Build history of the part. All positions in model axes, mm. Face numbers are marked on the shaded views. A direction names the side the tool comes from. Round coordinates to 2 decimals unless told otherwise and drop trailing zeros. Order: outer loops, then holes, each group sorted by start corner. A loop starts at its lowest first (then second) coordinate and runs counter-clockwise, first axis right, second up. Notation, with made-up numbers: M 50.25,11 L 97.25,11 A7 cw 97.25,16 Z; hole C 29,81 d5. An arc over 180 degrees is marked long. One line per item, written item: value. Start each with the question number.
Item 1: Band-saw the part on B-B, the plane y = -21.75. Write the cut outline in (x, z).
Item 2: Probe L1, parallel to X at y = -23.5, z = 0.7; L2, parallel to Y at x = 16.5, z = 0.6; L3, parallel to Y at x = 11, z = 0.35. List the from-to ranges inside material, lowest first.
Item 3: Band-saw the part on D-D, the plane x = 10.5. Write the cut outline in (y, z).
Item 4: Two-plate mould, pull along X, no slides. Class the marked faces 4, 5, 6 and 7: +X half, -X half, draft (parallel to the pull), parting line (faces both ways), or undercut.
Item 5: Tool access for the marked faces 1, 2 and 3: list every direction of +Z, -Z, +X, -X, +Y, -Y with a clear straight run to the whole face (end or side of a thin tool).
Item 6: Pin check, flat tips, straight feed: pin 1 (1 mm diameter, centred on x = 19, y = -35, fed in from -Z); pin 2 (2 mm diameter, centred on x = 12, y = -28.5, fed in from -Z); pin 3 (2 mm diameter, centred on y = -27.5, z = 0.5, fed in from -X). Stop position of each tip, or through.
Item 7: Band-saw the part on C-C, the plane x = 19. Write the cut outline in (y, z), then the cut area to 3 significant figures.
Item 8: Band-saw the part on A-A, the plane z = 0.8. Write the cut outline in (x, y).
Autodesk Inventor part; units mm, degrees
ref_plane "YZ Plane" through (0, 0, 0) normal (1, 0, 0) x (0, 1, 0)
ref_plane "XZ Plane" through (0, 0, 0) normal (0, 1, 0) x (-1, 0, 0)
ref_plane "XY Plane" through (0, 0, 0) normal (0, 0, 1) x (1, 0, 0)
ref_plane "Arbeitsebene1" through (0, 0, 0) normal (0, 0, 1) x (1, 0, 0)
sketch "Skizze1" plane through (0, 0, 0) normal (0, 0, 1) x (1, 0, 0)
  line L0 (8.8222, -7.25) -> (-9.1, -7.25)
  line L1 (-9.1, -7.25) -> (-9.1, 29.75)
  line L2 (-9.1, 29.75) -> (45.9, 29.75)
  line L3 (45.9, 29.75) -> (45.9, -7.25)
  line L4 (45.9, -7.25) -> (27.9778, -7.25)
  line L5 (-63.9, -32.5058) -> (-63.9, -38.75)
  line L6 (63.9, -38.75) -> (63.9, 3.9837)
  line L7 (63.9, 3.9837) -> (56.9, 3.9837)
  line L8 (56.9, 3.9837) -> (56.9, 8.0046)
  spline S0 degree 2 poles (56.9, 8.0046) (47.4544, 9.25) (56.9, 10.4954) knots 0.408689 0.408689 0.408689 2.009633 2.009633 2.009633 weights 1.06106 1.156332 1.06106
  line L9 (56.9, 10.4954) -> (56.9, 14.5163)
  line L10 (56.9, 14.5163) -> (63.9, 14.5163)
  arc A0 (63.9, 38.75) -> (59.9, 42.75) centre (59.9, 38.75) ccw
  line L11 (59.9, 42.75) -> (-59.9, 42.75)
  arc A1 (-59.9, 42.75) -> (-63.9, 38.75) centre (-59.9, 38.75) ccw
  line L12 (-63.9, 25.4963) -> (-55.9, 25.4963)
  line L13 (-55.9, 25.4963) -> (-55.9, 19.75)
  line L14 (-55.9, 19.75) -> (-18.9, 19.75)
  line L15 (-18.9, 19.75) -> (-18.9, 10.3274)
  spline S1 degree 2 poles (-18.9, 10.3274) (-11.6855, 9.25) (-18.9, 8.1726) knots 0.06387 0.06387 0.06387 0.952272 0.952272 0.952272 weights 1.010578 1.079212 1.010578
  line L16 (-18.9, 8.1726) -> (-18.9, -1.25)
  line L17 (-18.9, -1.25) -> (-55.9, -1.25)
  line L18 (-55.9, -1.25) -> (-55.9, -6.9963)
  line L19 (-55.9, -6.9963) -> (-63.9, -6.9963)
  line L20 (-63.9, -6.9963) -> (-63.9, -22.9942)
  line L21 (14.75, -32.05) -> (21.15, -32.05)
  line L22 (21.15, -32.05) -> (21.15, -24.25)
  line L23 (21.15, -24.25) -> (14.75, -24.25)
  line L24 (14.75, -24.25) -> (14.75, -32.05)
  line L25 (8.8222, -20.5) -> (30.4914, -20.5)
  line L26 (30.4914, -20.5) -> (30.4914, -39.25)
  line L27 (30.4914, -39.25) -> (8.8222, -39.25)
  line L28 (8.8222, -39.25) -> (8.8222, -20.5)
  line L29 (63.9, 14.5163) -> (63.9, 38.75)
  circle A2 centre (5.4922, -12.0867) radius 1.4
  circle A3 centre (17.95, -36.25) radius 1.4
  circle A4 centre (-27.8589, -14.9953) radius 1.4
  circle A5 centre (-42.2276, -36.25) radius 1.4
  circle A6 centre (-42.2276, -19.25) radius 1.4
  circle A7 centre (-27.8589, -39.949) radius 1.4
  circle A8 centre (27.4914, -28.65) radius 1.4
  circle A9 centre (32.285, -12.0867) radius 1.4
  line L30 (-8.36, -23.75) -> (8.8222, -23.75)
  line L31 (8.8222, -23.75) -> (8.8222, -7.25)
  line L32 (27.9778, -7.25) -> (27.9778, -25.25)
  line L33 (27.9778, -25.25) -> (21.15, -25.25)
  line L34 (21.15, -25.25) -> (21.15, -32.05)
  line L35 (21.15, -32.05) -> (14.75, -32.05)
  line L36 (14.75, -32.05) -> (14.75, -31.75)
  line L37 (14.75, -31.75) -> (-8.36, -31.75)
  line L38 (-8.36, -31.75) -> (-8.36, -36.25)
  line L39 (-8.36, -36.25) -> (-23.36, -36.25)
  line L40 (-23.36, -33.75) -> (-23.36, -36.25)
  line L41 (-38.36, -33.75) -> (-23.36, -33.75)
  line L42 (-38.36, -33.75) -> (-38.36, -31.25)
  line L43 (-38.36, -31.25) -> (-41.36, -31.25)
  line L44 (-41.36, -31.25) -> (-41.36, -32.5058)
  line L45 (-41.36, -32.5058) -> (-63.9, -32.5058)
  arc A10 (-63.9, -38.75) -> (-59.9, -42.75) centre (-59.9, -38.75) ccw
  line L46 (-59.9, -42.75) -> (59.9, -42.75)
  arc A11 (59.9, -42.75) -> (63.9, -38.75) centre (59.9, -38.75) ccw
  line L47 (-63.9, 38.75) -> (-63.9, 25.4963)
  line L48 (-63.9, -22.9942) -> (-41.36, -22.9942)
  line L49 (-41.36, -22.9942) -> (-41.36, -24.25)
  line L50 (-41.36, -24.25) -> (-38.36, -24.25)
  line L51 (-38.36, -24.25) -> (-38.36, -21.75)
  line L52 (-38.36, -21.75) -> (-23.36, -21.75)
  line L53 (-23.36, -19.25) -> (-23.36, -21.75)
  line L54 (-23.36, -19.25) -> (-8.36, -19.25)
  line L55 (-8.36, -19.25) -> (-8.36, -23.75)
  point P0 (0, 0)
  point P1 (15.25, -24.75)
  dimension "d0" = 0.5
extrude "Extrusion1" add sketch "Skizze1" along normal blind 4 contours L25 L32 L33 L22 L23 L24 L37 L28 | L25 L26 L27 L28 L37 L24 L21 L22 L33 L32 | L22 L21 L24 L23 | A3 | A8
sketch "Skizze2" plane through (0, 0, 0) normal (0, 0, -1) x (-1, 0, 0)
  line L0 (-8.8222, -39.25) -> (-30.4914, -39.25)
  line L1 (-8.8222, -20.5) -> (-8.8222, -39.25)
  line L2 (-30.4914, -20.5) -> (-8.8222, -20.5)
  line L3 (-30.4914, -39.25) -> (-30.4914, -20.5)
  line L4 (-14.75, -32.05) -> (-14.75, -24.25)
  line L5 (-8.8222, -20.5) -> (-8.8222, -39.25)
  line L6 (-14.75, -27.25) -> (-8.8222, -27.25)
  line L7 (-8.8222, -27.25) -> (-8.8222, -30.05)
  line L8 (-8.8222, -30.05) -> (-14.75, -30.05)
  line L9 (-14.75, -30.05) -> (-14.75, -27.25)
  line L10 (-14.75, -24.25) -> (-21.15, -24.25)
  line L11 (-30.4914, -20.5) -> (-8.8222, -20.5)
  line L12 (-19.35, -24.25) -> (-16.55, -24.25)
  line L13 (-16.55, -24.25) -> (-16.55, -20.5)
  line L14 (-16.55, -20.5) -> (-19.35, -20.5)
  line L15 (-19.35, -20.5) -> (-19.35, -24.25)
  point P0 (0, 0)
extrude "Extrusion2" cut sketch "Skizze2" against normal blind 2 contours L8 L4 L6 L1 | L2 L13 L10 L15
chamfer "Fase1" distance 1.8 angle 45 4 edges at (11.7861, -30.05, 0) (11.7861, -27.25, 0) (16.55, -22.375, 0) (19.35, -22.375, 0)
properties part number "20_Scanner_Fixation"
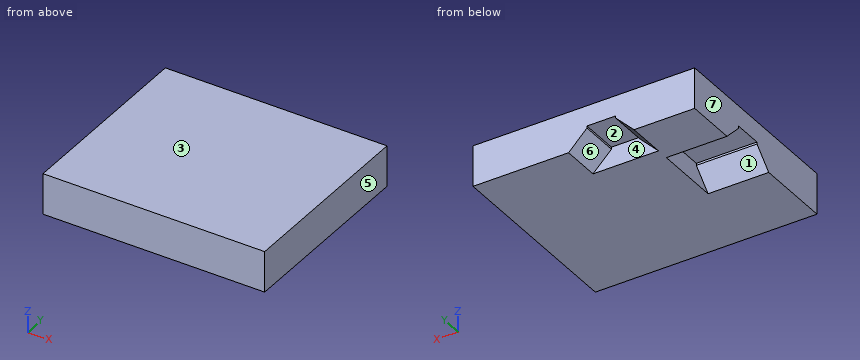
Output:
1. outline: M 8.82,0 L 14.75,0 L 16.55,1.8 L 16.55,2 L 19.35,2 L 19.35,1.8 L 21.15,0 L 30.49,0 L 30.49,4 L 8.82,4 Z
2. L1: x = 8.82 to 15.45, 20.45 to 30.49
2. L2: y = -39.25 to -24.25
2. L3: y = -39.25 to -31.5, -25.8 to -20.5
3. outline: M -39.25,0 L -31.85,0 L -30.05,1.8 L -30.05,2 L -27.25,2 L -27.25,1.8 L -25.45,0 L -20.5,0 L -20.5,4 L -39.25,4 Z
4. face 4: undercut
4. face 5: +X half
4. face 6: undercut
4. face 7: -X half
5. face 1: -Z, -X
5. face 2: -Z, +Y
5. face 3: +Z, +X, -X, +Y, -Y
6. pin 1: stops at z = 0
6. pin 2: stops at z = 2
6. pin 3: stops at x = 14.75
7. outline: M -39.25,0 L -24.25,0 L -24.25,2 L -20.5,2 L -20.5,4 L -39.25,4 Z
7. area: 67.5 mm²
8. outline: M 8.82,-39.25 L 30.49,-39.25 L 30.49,-20.5 L 20.35,-20.5 L 20.35,-24.25 L 15.55,-24.25 L 15.55,-20.5 L 8.82,-20.5 L 8.82,-26.25 L 14.75,-26.25 L 14.75,-31.05 L 8.82,-31.05 Z
